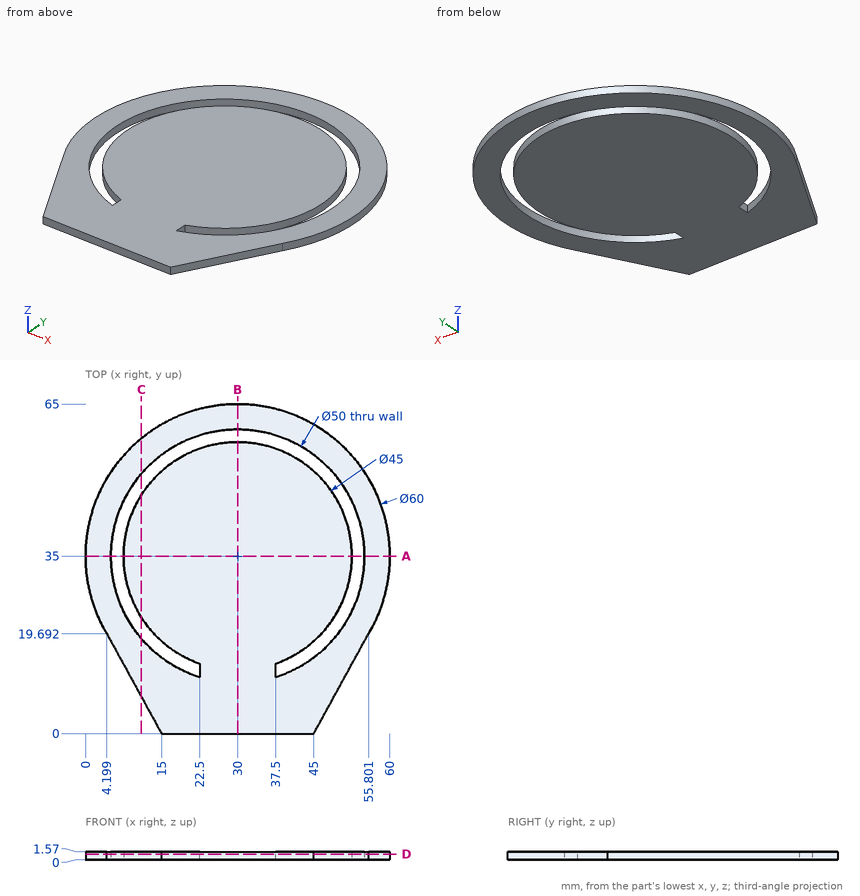
Geometry: see drawing. Coordinates: mm, zero at the bounding-box minimum. Coordinates: 2 decimals unless noted, no trailing zeros. Order: outer loops, then holes, each group sorted by start corner. A loop starts at its lowest first (then second) coordinate and runs counter-clockwise, first axis right, second up. Notation, with made-up numbers: M 14,-5.5 L 52,-5.5 A14 cw 52,16.5 Z; hole C 78,17.25 d7. An arc over 180 degrees is marked long. Write each question's results on one line, items separated by ' | '. Start each with the question number.
1) Section query C-C (x = 11). Return the cut outline in (y, z).
2) Section query B-B (x = 30). Return the cut outline in (y, z).
3) Section query A-A (y = 35). Return the cut outline in (x, z).
4) Contact query for flat-ended pins moving along their axis: pin 1 Ø0.8 at (y, z) = (13, 1) entering from +X; pin 2 Ø0.8 at (y, z) = (12, 1) entering from -X. Output: stop coordinate, or through.
5) Line query: line 1 (X direction, y = 35, z = 0.55); line 2 (X direction, y = 50, z = 1.05); line 3 (Y direction, x = 30, z = 1.15). Output: solid intervals per line, ascending. Write a range as from..to.
6) Section query D-D (z = 1.1). Return the cut outline in (x, y), plus the area to 3 significant figures.
Answers:
1) outline: M 7.29,0 L 18.75,0 L 18.75,1.57 L 7.29,1.57 Z; M 22.95,0 L 47.05,0 L 47.05,1.57 L 22.95,1.57 Z; M 51.25,0 L 58.22,0 L 58.22,1.57 L 51.25,1.57 Z
2) outline: M 0,0 L 57.5,0 L 57.5,1.57 L 0,1.57 Z; M 60,0 L 65,0 L 65,1.57 L 60,1.57 Z
3) outline: M 0,0 L 5,0 L 5,1.57 L 0,1.57 Z; M 7.5,0 L 52.5,0 L 52.5,1.57 L 7.5,1.57 Z; M 55,0 L 60,0 L 60,1.57 L 55,1.57 Z
4) pin 1: stops at x = 52.35 | pin 2: stops at x = 8.2
5) line 1: x = 0..5, 7.5..52.5, 55..60 | line 2: x = 4.02..10, 13.23..46.77, 50..55.98 | line 3: y = 0..57.5, 60..65
6) outline: M 4.2,19.69 L 15,0 L 45,0 L 55.8,19.69 A30 ccw long Z; hole M 22.5,11.15 L 22.5,13.79 A22.5 cw long 37.5,13.79 L 37.5,11.15 A25 ccw long Z | area: 2,760 mm^2
